```python
from build123d import *

# Parameters (mm, degrees)
SKETCH_2_W          = 16
SKETCH_2_H          = 12
SKETCH_2_R          = 0.933622945
EXTRUDE_1_DEPTH     = 1.5
SKETCH_3_W          = 8
SKETCH_3_H          = 2
EXTRUDE_2_DEPTH     = 7
SKETCH_4_R          = 1.5
CUT_EXTRUDE_1_DEPTH = 3


with BuildPart() as part:
    # 草图2 → 凸台-拉伸1 (new body)
    with BuildSketch(Plane.XY):
        with Locations((8, 6)):
            Rectangle(SKETCH_2_W, SKETCH_2_H)
        with Locations((2, 2.334057363)):
            Circle(SKETCH_2_R, mode=Mode.SUBTRACT)
        with Locations((14, 2.334057363)):
            Circle(SKETCH_2_R, mode=Mode.SUBTRACT)
    extrude(amount=EXTRUDE_1_DEPTH)

    # 草图3 → 凸台-拉伸2 (add)
    with BuildSketch(Plane.XY.offset(1.5)):
        with Locations((8, 11)):
            Rectangle(SKETCH_3_W, SKETCH_3_H)
    extrude(amount=EXTRUDE_2_DEPTH)

    # 草图4 → 切除-拉伸1 (cut)
    with BuildSketch(Plane.XZ.offset(-10)):
        with Locations((8, 4.86)):
            Circle(SKETCH_4_R)
    extrude(amount=-CUT_EXTRUDE_1_DEPTH, mode=Mode.SUBTRACT)


solid = part.part
```
The model under review builds one solid part; all positions refer to its coordinate system, in mm. A direction names the side the tool comes from. Give positions to 0.01 mm unless a question says otherwise; leave off trailing zeros. Write each loop counter-clockwise with the first axis right and the second up, starting at its lowest first coordinate (ties: lowest second). Pieces come first, ordered by that corner, then holes. Notation, with made-up numbers: M 37.5,36.25 L 66.5,36.25 A18 cw 66.5,47.25 Z; hole C 28.5,-27.5 d6. An arc over 180 degrees is marked long. Answer in a Markdown table with one row per item.
Item 1: Add section D-D on y = 8.5. Give the boundary of the cut face in (x, z).
Check sheet entries:
| item | result |
|---|---|
| outline | M 0,0 L 16,0 L 16,1.5 L 0,1.5 Z |
Item 2: For P1, Ø2.5, axis at x = 14, y = 2.33, coming from the +Z side; P2, Ø2, axis at y = 11, z = 4, coming from the -X side; P3, Ø1.6, axis at y = 11.5, z = 6, coming from the +X side, all flat-tipped, find the tip position at first contact; note any pin that passes through.
Check sheet entries:
| item | result |
|---|---|
| P1 | z = 1.5 |
| P2 | x = 4 |
| P3 | x = 12 |
Item 3: Add section A-A on x = 8. Give the boundary of the cut face in (y, z), plus the area to 3 significant figures.
Check sheet entries:
| item | result |
|---|---|
| outline | M 0,0 L 12,0 L 12,3.36 L 10,3.36 L 10,1.5 L 0,1.5 Z; M 10,6.36 L 12,6.36 L 12,8.5 L 10,8.5 Z |
| area | 26.0 mm2 |
Item 4: For line 1 along Y through (x, z) = (14, 0.65); line 2 along Z through (x, y) = (8, 10.5); line 3 along Z through (x, y) = (13, 1.25), list the stretches that pass through material, from the lowest coordinate up.
Check sheet entries:
| item | result |
|---|---|
| line 1 | 0 to 1.4, 3.27 to 12 |
| line 2 | 0 to 3.36, 6.36 to 8.5 |
| line 3 | 0 to 1.5 |
Item 5: Tool access review of faces 1 (the face through (8, 10, 7)), 2 (the face through (12, 11, 5)), 3 (the face through (8, 0, 1)): name each direction out of +Z, -Z, +X, -X, +Y, -Y from which nothing blocks a thin tool from reaching the whole face with its end or side.
Check sheet entries:
| item | result |
|---|---|
| face 1 | +Z, +X, -X, -Y |
| face 2 | +Z, +X, +Y, -Y |
| face 3 | +Z, -Z, +X, -X, -Y |
Item 6: Add section B-B on z = 4.86. Give the boundary of the cut face in (x, y), plus the area to 3 significant figures.
Check sheet entries:
| item | result |
|---|---|
| outline | M 4,10 L 6.5,10 L 6.5,12 L 4,12 Z; M 9.5,10 L 12,10 L 12,12 L 9.5,12 Z |
| area | 10.0 mm2 |
Item 7: Draft analysis for pull direction X (two halves, no side actions). For faces 4 (the face through (4, 11, 5)), 5 (the face through (6.89, 10.99, 5.87)), 6 (the face through (8, 6, 0)), state which applies: +X half, -X half, draft (parallel to the pull), parting line (faces both ways), or undercut.
Check sheet entries:
| item | result |
|---|---|
| face 4 | -X half |
| face 5 | undercut |
| face 6 | draft |
Item 8: Add section C-C on x = 14. Give the boundary of the cut face in (y, z).
Check sheet entries:
| item | result |
|---|---|
| outline | M 0,0 L 1.4,0 L 1.4,1.5 L 0,1.5 Z; M 3.27,0 L 12,0 L 12,1.5 L 3.27,1.5 Z |
